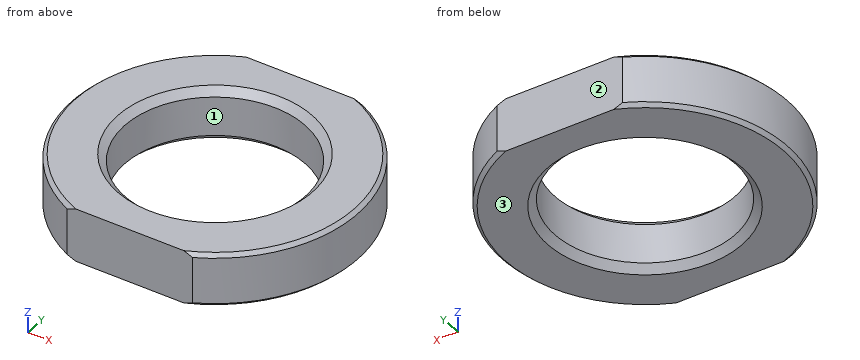
from build123d import *

# Parameters (mm, degrees)
SZKIC1_R                    = 40
DODANIE_WYCI_GNI_CIE1_DEPTH = 15
OTW_R_GWINTOWANY_M561_D     = 50.5
SFAZOWANIE1_SIZE            = 2
SFAZOWANIE2_SIZE            = 1
WYTNIJ_WYCI_GNI_CIE1_REACH  = 60.523
SZKIC4_W                    = 81.267228601
SZKIC4_H                    = 11.1112586


with BuildPart() as part:
    # Szkic1 → Dodanie-wyciągnięcie1 (new body)
    with BuildSketch(Plane.XY):
        Circle(SZKIC1_R)
    extrude(amount=DODANIE_WYCI_GNI_CIE1_DEPTH)

    # Otwór gwintowany M561 (through all)
    with Locations(Plane.XY.offset(15)):
        with Locations((0, 0)):
            Hole(OTW_R_GWINTOWANY_M561_D / 2)

    # Sfazowanie1
    sfazowanie1_edges = [part.edges().sort_by_distance(p)[0] for p in [
        (25.25, 0, 15),
        (25.25, 0, 0),
    ]]
    chamfer(sfazowanie1_edges, length=SFAZOWANIE1_SIZE)

    # Sfazowanie2
    sfazowanie2_edges = [part.edges().sort_by_distance(p)[0] for p in [
        (-40, 0, 0),
        (-40, 0, 15),
    ]]
    chamfer(sfazowanie2_edges, length=SFAZOWANIE2_SIZE)

    # Szkic4 → Wytnij-wyciągnięcie1 (cut, up to next)
    with BuildSketch(Plane.XY.offset(15), mode=Mode.PRIVATE) as wytnij_wyci_gni_cie1_sk1:
        with Locations((-4.392823168, -41.5556293)):
            Rectangle(SZKIC4_W, SZKIC4_H)
    wytnij_wyci_gni_cie1_tool1 = extrude(wytnij_wyci_gni_cie1_sk1.sketch, amount=-WYTNIJ_WYCI_GNI_CIE1_REACH, mode=Mode.PRIVATE) & part.part
    # Szkic4 → Wytnij-wyciągnięcie1 (cut, up to next)
    with BuildSketch(Plane.XY.offset(15), mode=Mode.PRIVATE) as wytnij_wyci_gni_cie1_sk2:
        with Locations((-4.392823168, 41.5556293)):
            Rectangle(SZKIC4_W, SZKIC4_H)
    wytnij_wyci_gni_cie1_tool2 = extrude(wytnij_wyci_gni_cie1_sk2.sketch, amount=-WYTNIJ_WYCI_GNI_CIE1_REACH, mode=Mode.PRIVATE) & part.part
    add(wytnij_wyci_gni_cie1_tool1.solids().sort_by_distance((-4.392823, -41.555629, 15))[0], mode=Mode.SUBTRACT)
    add(wytnij_wyci_gni_cie1_tool2.solids().sort_by_distance((-4.392823, 41.555629, 15))[0], mode=Mode.SUBTRACT)


solid = part.part
Could you check a few things on this model? Use its own coordinates, in mm. Face numbers are marked on the shaded views. Round coordinates to 2 decimals unless told otherwise and drop trailing zeros. Write each loop counter-clockwise with the first axis right and the second up, starting at its lowest first coordinate (ties: lowest second). Pieces come first, ordered by that corner, then holes. Notation, with made-up numbers: (-23.5, 9.25) - (23.5, 9.25) arc R21 cw to (23.5, 31.25) - close; hole circle Ø10 at (-2.75, 20.5). An arc over 180 degrees is marked (long way). Use a Markdown table: item, result.
Q1. I want a section at A-A (y = 0). List the corners of the cut face in (x, z) for me.
Output values:
| item | result |
|---|---|
| outline | (-40, 1) - (-39, 0) - (-27.25, 0) - (-25.25, 2) - (-25.25, 13) - (-27.25, 15) - (-39, 15) - (-40, 14) - close; (25.25, 2) - (27.25, 0) - (39, 0) - (40, 1) - (40, 14) - (39, 15) - (27.25, 15) - (25.25, 13) - close |
Q2. Please list where these lines run through material, in increasing order: L1, parallel to Y at x = 0, z = 8.5; L2, parallel to X at y = -9.5, z = 0.5; L3, parallel to X at y = -13.5, z = 3.5.
Output values:
| item | result |
|---|---|
| L1 | -36 to -25.25, 25.25 to 36 |
| L2 | -38.34 to -25.01, 25.01 to 38.34 |
| L3 | -37.65 to -21.34, 21.34 to 37.65 |
Q3. I want a section at B-B (x = 0). List the corners of the cut face in (y, z) for me, plus the area to 4 significant figures.
Output values:
| item | result |
|---|---|
| outline | (-36, 0) - (-27.25, 0) - (-25.25, 2) - (-25.25, 13) - (-27.25, 15) - (-36, 15) - close; (25.25, 2) - (27.25, 0) - (36, 0) - (36, 15) - (27.25, 15) - (25.25, 13) - close |
| area | 314.5 mm2 |
Q4. Thinking about a two-plate mould opening in Y: for the marked faces 1, 2 and 3, which applies, released by +Y, released by -Y, zero draft, split by the parting line, or undercut?
Output values:
| item | result |
|---|---|
| face 1 | undercut |
| face 2 | released by +Y |
| face 3 | zero draft |
Q5. For pin 1 (1.5 mm diameter, centred on y = 16.5, z = 13.5, fed in from +X); pin 2 (1.5 mm diameter, centred on y = -0.5, z = 11, fed in from -X); pin 3 (5 mm diameter, centred on y = 11.5, z = 5, fed in from +X); pin 4 (12 mm diameter, centred on x = -18.5, y = 13, fed in from +Z), each with a flat end and sliding along its axis, tell me the tip position at first contact or that it passes through.
Output values:
| item | result |
|---|---|
| pin 1 | x = 36.77 |
| pin 2 | x = -40 |
| pin 3 | x = 38.97 |
| pin 4 | z = 15 |
Q6. I want a section at C-C (z = 5). List the corners of the cut face in (x, y) for me.
Output values:
| item | result |
|---|---|
| outline | (-17.44, -36) - (17.44, -36) arc R40 ccw to (17.44, 36) - (-17.44, 36) arc R40 ccw to start; hole circle Ø50.5 at (0, 0) |
